For this review, use the dimensioned drawing (mm, ordinates from the lowest corner) and the shaded views. Coordinates: 2 decimals unless noted, no trailing zeros. Loops run counter-clockwise (first coordinate to the right, second up) from the corner with the lowest first, then second, coordinate; pieces in that order, holes last. Notation, with made-up numbers: M 31.5,-14.75 L 65.5,-14.75 A21 cw 65.5,5.25 Z; hole C 29.25,34 d1. An arc over 180 degrees is marked long. Write item = value, one per line. Start each with the question number.
Q1. We need section B-B on z = 15. Give the boundary of the cut face in (x, y).
Q2. Mouldability with a two-part tool opening along X and no side actions: class the marked faces 1, 2 and 3 as released by +X, released by -X, zero draft, split by the parting line, or undercut.
Q3. Wall thickness on probe 1 along Y at (x, z) = (6.35, 34.5); probe 2 along X at (y, z) = (7.75, 28) (1 decimal); probe 3 along Y at (x, z) = (6.5, 2): over which ranges is each line inside the solid? List them lowest first.
Q4. Clearance check with flat-ended pins moving along their axes: pin 1 Ø1.5 at (y, z) = (10, 34) entering from +X; pin 2 Ø2 at (x, z) = (2, 15) entering from +Y (1 decimal); pin 3 Ø1 at (x, z) = (8, 32) entering from -Y (1 decimal). State where each tip first meets the part, or that it passes through.
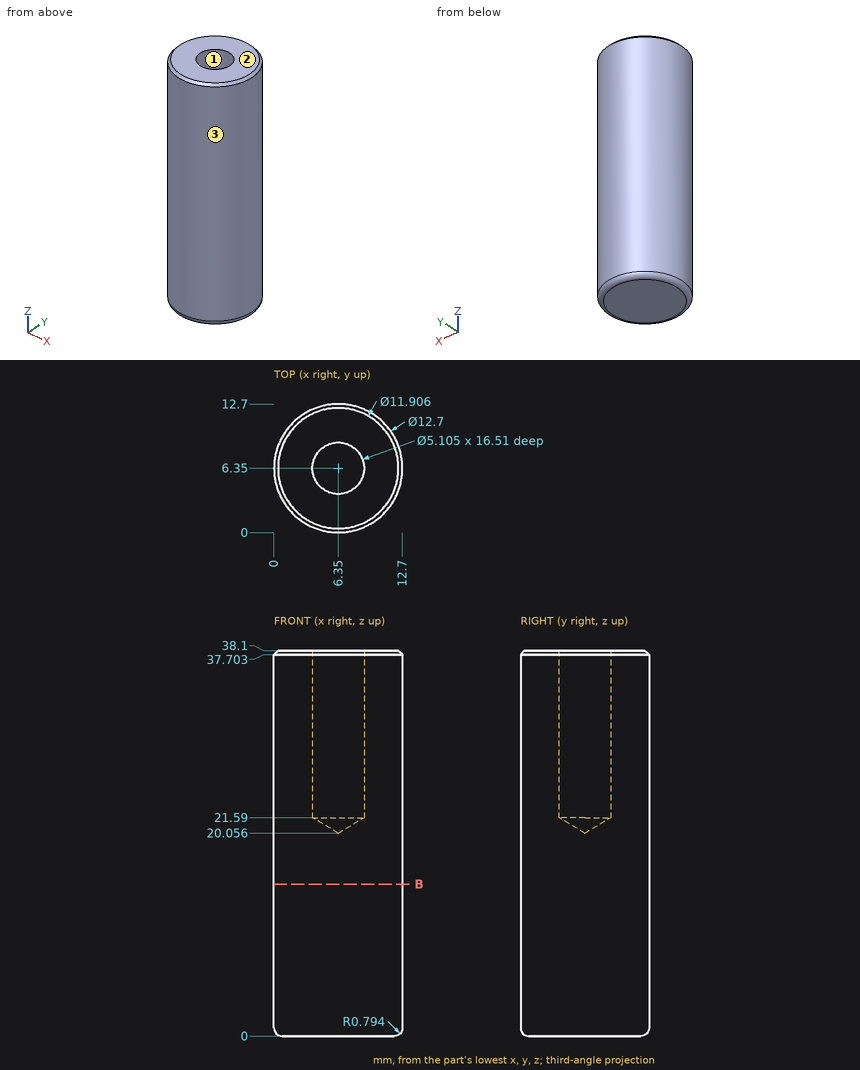
Returned:
q1.outline = C 6.35,6.35 d12.7
q2.face_1 = undercut
q2.face_2 = zero draft
q2.face_3 = split by the parting line
q3.probe_1 = 0 to 3.8, 8.9 to 12.7
q3.probe_2 = 0.2 to 4.2, 8.5 to 12.5
q3.probe_3 = 0 to 12.7
q4.pin_1 = 12
q4.pin_2 = 11.7
q4.pin_3 = 0.1
